Solid Edge part; units mm, degrees
sketch "Sketch1" plane through (0, 0, 0) normal (0, 0, 1) x (1, 0, 0)
  line L0 (-22.5, -25) -> (22.5, -25)
  line L1 (22.5, -25) -> (22.5, 25)
  line L2 (22.5, 25) -> (-22.5, 25)
  line L3 (-22.5, 25) -> (-22.5, -25)
  dimension "D1" = 22.5
  dimension "D2" = 22.5
extrude "Protrusion1" add sketch "Sketch1" along normal blind 1
hole "Hole_1" at (-18.5, 21, 1) direction (0, 0, -1) diameter 3.2 end up to next
hole "Hole1" at (18.5, 21, 1) direction (0, 0, -1) diameter 3.2 end up to next
hole "Hole2" at (18.5, -21, 1) direction (0, 0, -1) diameter 3.2 end up to next
hole "Hole3" at (-18.5, -21, 1) direction (0, 0, -1) diameter 3.2 end up to next
properties material "Polyethylene, low density"
Read the model definition and answer for the solid it produces. Units are mm, in the model's axes. Give positions to 0.01 mm unless a question says otherwise; leave off trailing zeros. Loops run counter-clockwise (first coordinate to the right, second up) from the corner with the lowest first, then second, coordinate; pieces in that order, holes last. Notation, with made-up numbers: (-23.5, 71.5) -> (23.5, 71.5) arc R27 ccw to (23.5, 108.5) -> close; hole circle Ø5 at (-36.75, 26.5). An arc over 180 degrees is marked (long way). Use a Markdown table: item, result.
Q1. Find the intervals of material crossed by line 1 along X through (y, z) = (21, 0.2); line 2 along Y through (x, z) = (18.5, 0.7); line 3 along X through (y, z) = (-20, 0.5), in increasing order.
Solved:
| item | result |
|---|---|
| line 1 | x = -22.5 to -20.1, -16.9 to 16.9, 20.1 to 22.5 |
| line 2 | y = -25 to -22.6, -19.4 to 19.4, 22.6 to 25 |
| line 3 | x = -22.5 to -19.75, -17.25 to 17.25, 19.75 to 22.5 |
Q2. Section B-B, the plane x = 18.5 is taken. Determine the outline of the cut face in (y, z), then the cut area to 3 significant figures.
Solved:
| item | result |
|---|---|
| outline | (-25, 0) -> (-22.6, 0) -> (-22.6, 1) -> (-25, 1) -> close; (-19.4, 0) -> (19.4, 0) -> (19.4, 1) -> (-19.4, 1) -> close; (22.6, 0) -> (25, 0) -> (25, 1) -> (22.6, 1) -> close |
| area | 43.6 mm^2 |
Q3. Section A-A, the plane y = -21 is taken. Determine the outline of the cut face in (x, z).
Solved:
| item | result |
|---|---|
| outline | (-22.5, 0) -> (-20.1, 0) -> (-20.1, 1) -> (-22.5, 1) -> close; (-16.9, 0) -> (16.9, 0) -> (16.9, 1) -> (-16.9, 1) -> close; (20.1, 0) -> (22.5, 0) -> (22.5, 1) -> (20.1, 1) -> close |
Q4. Determine the mould class of faces 1 (the face through (0, 0, 1)), 2 (the face through (-16.914, 21.208, 0.507)) for opening direction Y: pulls with the +Y half, pulls with the -Y half, needs draft (parallel to the pull), parting line crosses it, or undercut.
Solved:
| item | result |
|---|---|
| face 1 | needs draft |
| face 2 | undercut |
